CAD build for the part. Positions are in the model's coordinates, mm. A direction names the side the tool comes from. Give positions to 0.01 mm unless a question says otherwise; leave off trailing zeros. Write each loop counter-clockwise with the first axis right and the second up, starting at its lowest first coordinate (ties: lowest second). Pieces come first, ordered by that corner, then holes. Notation, with made-up numbers: (5.5, 52.25) - (45.5, 52.25) arc R24 cw to (45.5, 68.25) - close; hole circle Ø6 at (-24.5, 88). An arc over 180 degrees is marked (long way). Put each result on its own line as item: value. Start each with the question number.
1. Cut at B-B on z = -4.25. List the corners of the cut face in (x, y), and give its area (3 significant figures).
2. Mould opens along Z. For faces 1 (the cylindrical face through (-2.77, 3.94, -3.61)), 2 (the flat face through (-2, 0, 2)), 3 (the flat face through (3.13, 13.8, -3.25)) say: +Z half, -Z half, draft (parallel to the pull), parting line (faces both ways), or undercut.
3. Tool access for faces 4 (the flat face through (-1.178, 13.802, 4.385)), 5 (the flat face through (-2.24, 13.8, -3.79)), 6 (the flat face through (-4, 8, 3)): list every direction of +Z, -Z, +X, -X, +Y, -Y with a clear straight run to the whole face (end or side of a thin tool).
4. Wall check: line 1 (Y direction, x = 0.5, z = 4.75); line 2 (Y direction, x = -0.5, z = -4); line 3 (X direction, y = 18.3, z = 0). Give the ranges that are in metal, low to high.
5. Cut at D-D on x = 3.25. List the corners of the cut face in (y, z).
6. Drop flat-ended pins along their axis: pin 1 (3 mm diameter, centred on y = 5.5, z = 3, fed in from -X); pin 2 (4 mm diameter, centred on x = -4.5, y = 10.5, fed in from +Z); pin 3 (5.5 mm diameter, centred on y = 14, z = 0, fed in from +X); pin 4 (4 mm diameter, centred on x = 0, z = 0, fed in from -Y). Give the stop position or say it passes through.
7. Cut at A-A on z = 0. List the corners of the cut face in (x, y).
8. Cut at C-C on y = 6.25. List the corners of the cut face in (x, z).
from build123d import *

# Parameters (mm, degrees)
SKETCH1_R           = 4.55
BOSS_EXTRUDE1_DEPTH = 8
SKETCH2_R           = 2.5
CUT_EXTRUDE1_DEPTH  = 8
SKETCH3_R           = 6.5
BOSS_EXTRUDE4_DEPTH = 9.5
CUT_EXTRUDE2_DEPTH  = 7.5
SKETCH6_R           = 6.5
BOSS_EXTRUDE5_DEPTH = 2
SKETCH7_R           = 2.5
CUT_EXTRUDE3_DEPTH  = 22.558061137


with BuildPart() as part:
    # Sketch1 → Boss-Extrude1 (new body)
    with BuildSketch(Plane(origin=(0, 0, 0), x_dir=(1, 0, 0), z_dir=(0, 1, 0))):
        with Locations(Location((0, 0, 0), (0, 0, 270))):
            Circle(SKETCH1_R)
    extrude(amount=BOSS_EXTRUDE1_DEPTH)

    # Sketch2 → Cut-Extrude1 (cut)
    with BuildSketch(Plane(origin=(0, 8, 0), x_dir=(1, 0, 0), z_dir=(0, 1, 0))):
        with Locations(Location((0, 0, 0), (0, 0, 270))):
            Circle(SKETCH2_R)
    extrude(amount=-CUT_EXTRUDE1_DEPTH, mode=Mode.SUBTRACT)

    # Sketch3 → Boss-Extrude4 (add)
    with BuildSketch(Plane(origin=(0, 8, 0), x_dir=(1, 0, 0), z_dir=(0, 1, 0))):
        with Locations(Location((0, 0, 0), (0, 0, 270))):
            Circle(SKETCH3_R)
    extrude(amount=BOSS_EXTRUDE4_DEPTH)

    # Sketch5 → Cut-Extrude2 (cut)
    with BuildSketch(Plane(origin=(0, 17.5, 0), x_dir=(1, 0, 0), z_dir=(0, 1, 0))):
        Polygon((-4.406153459, -2.521016119), (-4.406153459, 2.55966625), (-0.006153459, 5.061357304), (7.819258761, 0.543353452), (3.435994759, -7.048682503), align=None)
    extrude(amount=-CUT_EXTRUDE2_DEPTH, mode=Mode.SUBTRACT)

    # Sketch6 → Boss-Extrude5 (add)
    with BuildSketch(Plane(origin=(0, 17.5, 0), x_dir=(1, 0, 0), z_dir=(0, 1, 0))):
        with Locations(Location((0, 0, 0), (0, 0, 270))):
            Circle(SKETCH6_R)
    extrude(amount=BOSS_EXTRUDE5_DEPTH)

    # Sketch7 → Cut-Extrude3 (cut, through all)
    with BuildSketch(Plane.XZ):
        with Locations(Location((0, 0, 0), (0, 0, 90))):
            Circle(SKETCH7_R)
    extrude(amount=-CUT_EXTRUDE3_DEPTH, mode=Mode.SUBTRACT)


solid = part.part
Report:
1. outline: (-4.92, 8) - (-1.62, 8) - (-1.62, 0) - (1.62, 0) - (1.62, 8) - (4.92, 8) - (4.92, 19.5) - (-4.92, 19.5) - close; hole (-1.43, 10) - (1.4, 10) - (1.4, 17.5) - (-1.43, 17.5) - close
1. area: 118 mm²
2. face 1: parting line
2. face 2: draft
2. face 3: undercut
3. face 4: +X
3. face 5: none
3. face 6: -Y
4. line 1: y = 8 to 10, 17.5 to 19.5
4. line 2: y = 0 to 10, 17.5 to 19.5
4. line 3: x = -6.5 to -2.5, 2.5 to 6.5
5. outline: (0, -3.18) - (8, -3.18) - (8, -5.63) - (19.5, -5.63) - (19.5, 5.63) - (17.5, 5.63) - (17.5, -3.18) - (10, -3.18) - (10, 5.63) - (8, 5.63) - (8, 3.18) - (0, 3.18) - close
6. pin 1: stops at x = -4.3
6. pin 2: stops at z = 6
6. pin 3: stops at x = 6.35
6. pin 4: passes through
7. outline: (-6.5, 8) - (-4.55, 8) - (-4.55, 0) - (-2.5, 0) - (-2.5, 10) - (-4.41, 10) - (-4.41, 17.5) - (-2.5, 17.5) - (-2.5, 19.5) - (-6.5, 19.5) - close; (2.5, 0) - (4.55, 0) - (4.55, 8) - (6.5, 8) - (6.5, 10) - (2.5, 10) - close; (2.5, 17.5) - (6.5, 17.5) - (6.5, 19.5) - (2.5, 19.5) - close
8. outline: circle Ø9.1 at (0, 0); hole circle Ø5 at (0, 0)
